Check sheet for the modelled part. Datum: model origin and axes. Units: mm. A direction names the side the tool comes from. Coordinates: 2 decimals unless noted, no trailing zeros. Loops run counter-clockwise (first coordinate to the right, second up) from the corner with the lowest first, then second, coordinate; pieces in that order, holes last. Notation, with made-up numbers: M 41.25,-6.5 L 79.25,-6.5 A23 ccw 79.25,27.5 Z; hole C 19.25,9 d10. An arc over 180 degrees is marked long. Answer as CSV lines item,"result". Start each with the question number.
from build123d import *

# Parameters (mm, degrees)
F0_W     = 2000
F0_H     = 1000
F0_W_2   = 1800
F0_H_2   = 800
F1_DEPTH = 2000
F3_DEPTH = 2225.647926
F4_DEPTH = 1010.152698


with BuildPart() as f1:
    # F0 (on Top) → F1 (new body)
    with BuildSketch(Plane.XY):
        Rectangle(F0_W, F0_H)
        Rectangle(F0_W_2, F0_H_2, mode=Mode.SUBTRACT)
    extrude(amount=F1_DEPTH)

    # F2 (on face) → F3 (cut)
    with BuildSketch(Plane.XZ.offset(500)):
        with BuildLine():
            ThreePointArc((-495.205782, 1600.000029), (-559.896999, 1696.817267), (-674.100717, 1674.100717))
            Line((-674.100717, 1674.100717), (-525.899312, 1525.899312))
            ThreePointArc((-525.899312, 1525.899312), (-503.182771, 1559.897009), (-495.205782, 1600.000029))
        make_face()
        with BuildLine():
            ThreePointArc((674.100702, 1674.100702), (525.899298, 1674.100702), (525.899298, 1525.899298))
            Line((525.899298, 1525.899298), (674.100702, 1674.100702))
        make_face()
        with BuildLine():
            Line((674.100702, 1674.100702), (525.899298, 1525.899298))
            ThreePointArc((525.899298, 1525.899298), (640.103011, 1503.182767), (704.794218, 1600))
            ThreePointArc((704.794218, 1600), (696.817233, 1640.103011), (674.100702, 1674.100702))
        make_face()
        with BuildLine():
            ThreePointArc((704.794218, 400), (640.103011, 496.817233), (525.899298, 474.100702))
            Line((525.899298, 474.100702), (674.100702, 325.899298))
            ThreePointArc((674.100702, 325.899298), (696.817233, 359.896989), (704.794218, 400))
        make_face()
        with BuildLine():
            Line((674.100702, 325.899298), (525.899298, 474.100702))
            ThreePointArc((525.899298, 474.100702), (525.899298, 325.899298), (674.100702, 325.899298))
        make_face()
        with BuildLine():
            ThreePointArc((-495.205782, 400.000029), (-503.182763, 440.103031), (-525.899283, 474.100717))
            Line((-525.899283, 474.100717), (-674.100688, 325.899312))
            ThreePointArc((-674.100688, 325.899312), (-559.896979, 303.1828), (-495.205782, 400.000029))
        make_face()
        with BuildLine():
            Line((-674.100688, 325.899312), (-525.899283, 474.100717))
            ThreePointArc((-525.899283, 474.100717), (-674.100702, 474.100732), (-674.100688, 325.899312))
        make_face()
        with BuildLine():
            ThreePointArc((176.776695, 1176.776695), (0, 1250), (-176.776695, 1176.776695))
            Line((-176.776695, 1176.776695), (0, 1000))
            Line((0, 1000), (176.776695, 1176.776695))
        make_face()
        with BuildLine():
            Line((0, 1000), (-176.776695, 1176.776695))
            ThreePointArc((-176.776695, 1176.776695), (-250, 1000), (-176.776695, 823.223305))
            Line((-176.776695, 823.223305), (0, 1000))
        make_face()
        with BuildLine():
            Line((-525.899312, 1525.899312), (-674.100717, 1674.100717))
            ThreePointArc((-674.100717, 1674.100717), (-674.100702, 1525.899327), (-525.899312, 1525.899312))
        make_face()
        with BuildLine():
            Line((176.776695, 1176.776695), (0, 1000))
            Line((0, 1000), (176.776695, 823.223305))
            ThreePointArc((176.776695, 823.223305), (230.969883, 904.329142), (250, 1000))
            ThreePointArc((250, 1000), (230.969883, 1095.670858), (176.776695, 1176.776695))
        make_face()
        with BuildLine():
            Line((176.776695, 823.223305), (0, 1000))
            Line((0, 1000), (-176.776695, 823.223305))
            ThreePointArc((-176.776695, 823.223305), (0, 750), (176.776695, 823.223305))
        make_face()
    extrude(amount=-F3_DEPTH, mode=Mode.SUBTRACT)

    # F2 (on face) → F4 (cut)
    with BuildSketch(Plane.XZ.offset(500)):
        with BuildLine():
            ThreePointArc((-495.205782, 1600.000029), (-559.896999, 1696.817267), (-674.100717, 1674.100717))
            Line((-674.100717, 1674.100717), (-525.899312, 1525.899312))
            ThreePointArc((-525.899312, 1525.899312), (-503.182771, 1559.897009), (-495.205782, 1600.000029))
        make_face()
        with BuildLine():
            ThreePointArc((674.100702, 1674.100702), (525.899298, 1674.100702), (525.899298, 1525.899298))
            Line((525.899298, 1525.899298), (674.100702, 1674.100702))
        make_face()
        with BuildLine():
            Line((674.100702, 1674.100702), (525.899298, 1525.899298))
            ThreePointArc((525.899298, 1525.899298), (640.103011, 1503.182767), (704.794218, 1600))
            ThreePointArc((704.794218, 1600), (696.817233, 1640.103011), (674.100702, 1674.100702))
        make_face()
        with BuildLine():
            ThreePointArc((704.794218, 400), (640.103011, 496.817233), (525.899298, 474.100702))
            Line((525.899298, 474.100702), (674.100702, 325.899298))
            ThreePointArc((674.100702, 325.899298), (696.817233, 359.896989), (704.794218, 400))
        make_face()
        with BuildLine():
            Line((674.100702, 325.899298), (525.899298, 474.100702))
            ThreePointArc((525.899298, 474.100702), (525.899298, 325.899298), (674.100702, 325.899298))
        make_face()
        with BuildLine():
            ThreePointArc((-495.205782, 400.000029), (-503.182763, 440.103031), (-525.899283, 474.100717))
            Line((-525.899283, 474.100717), (-674.100688, 325.899312))
            ThreePointArc((-674.100688, 325.899312), (-559.896979, 303.1828), (-495.205782, 400.000029))
        make_face()
        with BuildLine():
            Line((-674.100688, 325.899312), (-525.899283, 474.100717))
            ThreePointArc((-525.899283, 474.100717), (-674.100702, 474.100732), (-674.100688, 325.899312))
        make_face()
        with BuildLine():
            ThreePointArc((176.776695, 1176.776695), (0, 1250), (-176.776695, 1176.776695))
            Line((-176.776695, 1176.776695), (0, 1000))
            Line((0, 1000), (176.776695, 1176.776695))
        make_face()
        with BuildLine():
            Line((0, 1000), (-176.776695, 1176.776695))
            ThreePointArc((-176.776695, 1176.776695), (-250, 1000), (-176.776695, 823.223305))
            Line((-176.776695, 823.223305), (0, 1000))
        make_face()
        with BuildLine():
            Line((-525.899312, 1525.899312), (-674.100717, 1674.100717))
            ThreePointArc((-674.100717, 1674.100717), (-674.100702, 1525.899327), (-525.899312, 1525.899312))
        make_face()
        with BuildLine():
            Line((176.776695, 1176.776695), (0, 1000))
            Line((0, 1000), (176.776695, 823.223305))
            ThreePointArc((176.776695, 823.223305), (230.969883, 904.329142), (250, 1000))
            ThreePointArc((250, 1000), (230.969883, 1095.670858), (176.776695, 1176.776695))
        make_face()
        with BuildLine():
            Line((176.776695, 823.223305), (0, 1000))
            Line((0, 1000), (-176.776695, 823.223305))
            ThreePointArc((-176.776695, 823.223305), (0, 750), (176.776695, 823.223305))
        make_face()
    extrude(amount=-F4_DEPTH, mode=Mode.SUBTRACT)


solid = f1.part
Item 1: Material ranges on line 1 (X direction, y = 47, z = 261.5); line 2 (Y direction, x = -522, z = 684.5); line 3 (X direction, y = 442.5, z = 331.5), recorded low to high. Write a range as from..to.
Item 2: Sectioned sample at D-D, the plane z = 1798. Record the boundary of the cut face in (x, y), and give its area (3 significant figures).
Item 3: Sectioned sample at A-A, the plane y = 287. Record the boundary of the cut face in (x, z).
Item 4: Release check for a two-part mould opening along Y. For faces 1 (the face through (-236, -500, 764)), 2 (the face through (-900, -6, 986)), 3 (the face through (-79, -405, 2000)) record: released by +Y, released by -Y, zero draft, split by the parting line, or undercut.
Item 5: Sectioned sample at C-C, the plane x = -600. Record the boundary of the cut face in (y, z), and give its area (3 significant figures).
Item 6: Sectioned sample at B-B, the plane x = 328. Record the boundary of the cut face in (y, z), and give its area (3 significant figures).
Item 7: Set-up check for faces 4 (the face through (-1000, -7, 986)), 5 (the face through (-213, 400, 764)): record each of +Z, -Z, +X, -X, +Y, -Y from which the full face is reachable in a straight line by a thin tool's end or side.
Reply:
1,line 1,"-1000..-900, 900..1000"
1,line 2,"-500..-400, 400..500"
1,line 3,"-1000..-679.31, -520.69..520.69, 679.31..1000"
2,outline,"M -1000,-500 L 1000,-500 L 1000,500 L -1000,500 Z; hole M -900,-400 L 900,-400 L 900,400 L -900,400 Z"
2,area,"560,000 mm²"
3,outline,"M -1000,0 L -900,0 L -900,2000 L -1000,2000 Z; M 900,0 L 1000,0 L 1000,2000 L 900,2000 Z"
4,face 1,"released by -Y"
4,face 2,"undercut"
4,face 3,"zero draft"
5,outline,"M -500,0 L -400,0 L -400,295.21 L -500,295.21 Z; M -500,504.79 L -400,504.79 L -400,1495.21 L -500,1495.21 Z; M -500,1704.79 L -400,1704.79 L -400,2000 L -500,2000 Z; M 400,0 L 500,0 L 500,295.21 L 400,295.21 Z; M 400,504.79 L 500,504.79 L 500,1495.21 L 400,1495.21 Z; M 400,1704.79 L 500,1704.79 L 500,2000 L 400,2000 Z"
5,area,"316,000 mm²"
6,outline,"M -500,0 L -400,0 L -400,2000 L -500,2000 Z; M 400,0 L 500,0 L 500,2000 L 400,2000 Z"
6,area,"400,000 mm²"
7,face 4,"+Z, -Z, -X, +Y, -Y"
7,face 5,"+Z, -Z"
